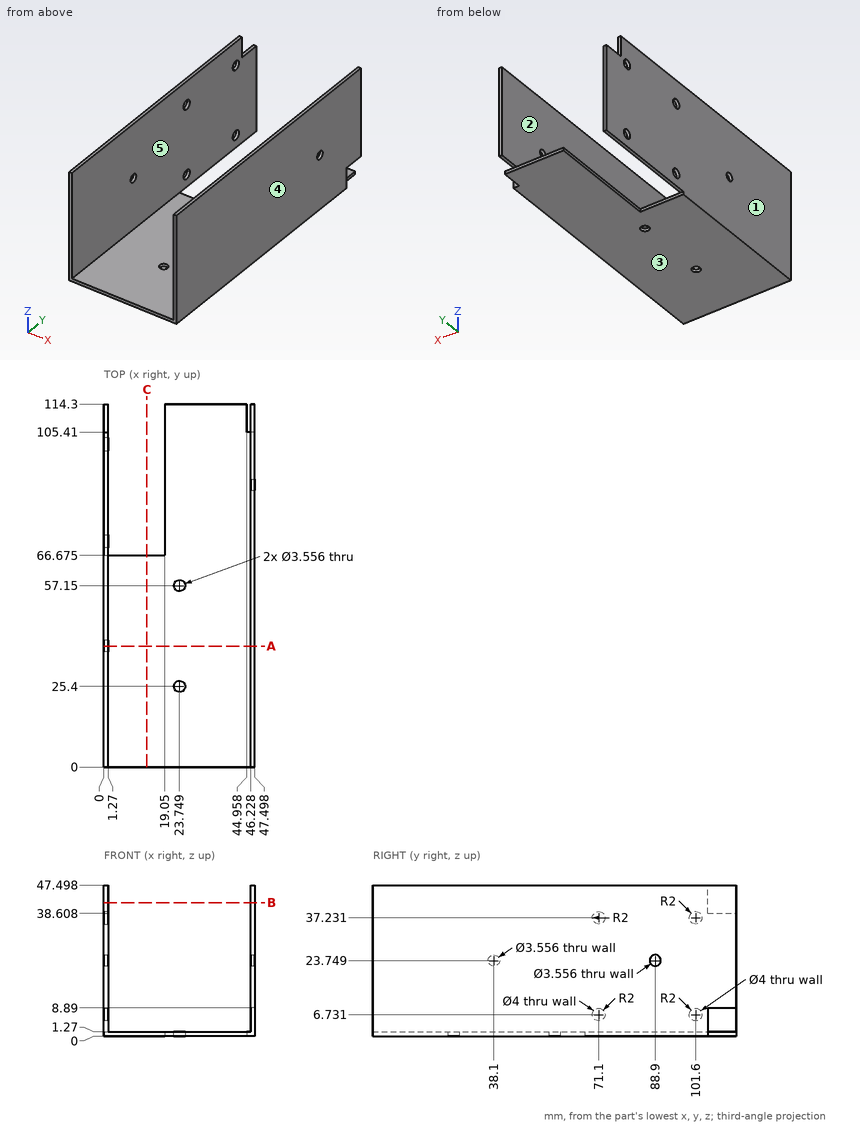
Answer from the drawing. Dimensions are ordinates in mm from the lowest x, y and z of the part. A direction names the side the tool comes from. Round coordinates to 2 decimals unless told otherwise and drop trailing zeros. Loops run counter-clockwise (first coordinate to the right, second up) from the corner with the lowest first, then second, coordinate; pieces in that order, holes last.
(1) The part is cut by section C-C, the plane x = 13.5. Give the vertices of the cut face in (y, z) (3 decimals).
Computed values:
outline: (0, 0) - (66.675, 0) - (66.675, 1.27) - (0, 1.27) - close
(2) Find the intervals of material crossed by L1, parallel to Z at x = 0.6, y = 71.1; L2, parallel to X at y = 10, z = 35.5; L3, parallel to Z at x = 47.1, y = 88.9, in increasing order.
Computed values:
L1: z = 1.27 to 4.73, 8.73 to 35.23, 39.23 to 47.5
L2: x = 0 to 1.27, 46.23 to 47.5
L3: z = 0 to 21.97, 25.53 to 47.5
(3) The part is cut by section B-B, the plane z = 42. Give the vertices of the cut face in (x, y), and give its area (3 significant figures).
Computed values:
outline: (0, 0) - (1.27, 0) - (1.27, 105.41) - (0, 105.41) - close; (46.23, 0) - (47.5, 0) - (47.5, 114.3) - (46.23, 114.3) - close
area: 279 mm2
(4) The mould has two halves that part along X. Classify the marked faces 1, 2 and 3: pulls with the +X half, pulls with the -X half, needs draft (parallel to the pull), parting line crosses it, or undercut.
Computed values:
face 1: pulls with the -X half
face 2: undercut
face 3: needs draft
(5) The part is cut by section A-A, the plane y = 38.1. Give the vertices of the cut face in (x, z), and give its area (3 significant figures).
Computed values:
outline: (0, 0) - (47.5, 0) - (47.5, 47.5) - (46.23, 47.5) - (46.23, 1.27) - (1.27, 1.27) - (1.27, 21.97) - (0, 21.97) - close; (0, 25.53) - (1.27, 25.53) - (1.27, 47.5) - (0, 47.5) - close
area: 173 mm2
(6) For the marked faces 4 and 5, determine the directions among +Z, -Z, +X, -X, +Y, -Y from which every point of the face is accessible in a straight line to the end or side of a thin tool.
Computed values:
face 4: +Z, -Z, +X, +Y, -Y
face 5: +Z, +Y, -Y
(7) Each of these flat-tipped pins is pushed along its axis until it touches: P1, Ø1.4, axis at x = 8, z = 1, coming from the +Y side (3 decimals); P2, Ø12, axis at x = 23, z = 10, coming from the -Y side; P3, Ø3, axis at x = 46.5, z = 3, coming from the +Y side; P4, Ø3, axis at y = 101.6, z = 6.731, coming from the -X side. Where does it stop, or does it pass through?
Computed values:
P1: stops at y = 66.675
P2: passes through
P3: stops at y = 105.41
P4: stops at x = 46.23
